```python
from build123d import *

# Parameters (mm, degrees)
EXTRUDE_THIN1_DEPTH = 9.525
FILLET1_R           = 1
FILLET3_R           = 2
FILLET4_R           = 2
SKETCH2_R           = 2.2
CUT_EXTRUDE1_DEPTH  = 23.468607993
CUT_EXTRUDE2_REACH  = 24.469
SKETCH3_R           = 1.7525


with BuildPart() as part:
    # Sketch1 → Extrude-Thin1 (new body)
    with BuildSketch(Plane(origin=(0, 0, 0), x_dir=(1, 0, 0), z_dir=(0, 1, 0))):
        Polygon((0, 0), (0, -15.9004), (12.7, -15.9004), (12.7, 0), (11.1125, 0), (11.1125, -14.3129), (1.5875, -14.3129), (1.5875, 0), align=None)
    extrude(amount=EXTRUDE_THIN1_DEPTH)

    # Fillet1
    fillet1_edges = [part.edges().sort_by_distance(p)[0] for p in [
        (1.5875, 4.7625, 14.3129),
        (11.1125, 4.7625, 14.3129),
    ]]
    fillet(fillet1_edges, radius=FILLET1_R)

    # Fillet3
    fillet3_edges = [part.edges().sort_by_distance(p)[0] for p in [
        (12.7, 4.7625, 15.9004),
        (0, 4.7625, 15.9004),
    ]]
    fillet(fillet3_edges, radius=FILLET3_R)

    # Fillet4
    fillet4_edges = [part.edges().sort_by_distance(p)[0] for p in [
        (0.79375, 9.525, 0),
        (0.79375, 0, 0),
        (11.90625, 9.525, 0),
        (11.90625, 0, 0),
    ]]
    fillet(fillet4_edges, radius=FILLET4_R)

    # Sketch2 → Cut-Extrude1 (cut, through all)
    with BuildSketch(Plane.ZY):
        with Locations((4.7625, 4.7625)):
            Circle(SKETCH2_R)
    extrude(amount=-CUT_EXTRUDE1_DEPTH, mode=Mode.SUBTRACT)

    # Sketch3 → Cut-Extrude2 (cut, up to next)
    with BuildSketch(Plane.XY.offset(15.9004), mode=Mode.PRIVATE) as cut_extrude2_sk1:
        with Locations((6.35, 4.7625)):
            Circle(SKETCH3_R)
    cut_extrude2_tool1 = extrude(cut_extrude2_sk1.sketch, amount=-CUT_EXTRUDE2_REACH, mode=Mode.PRIVATE) & part.part
    add(cut_extrude2_tool1.solids().sort_by_distance((6.35, 4.7625, 15.9004))[0], mode=Mode.SUBTRACT)


solid = part.part
```
Here's how the part is built. I have some questions about the finished solid (model axes, mm). A direction names the side the tool comes from. Coordinates: 2 decimals unless noted, no trailing zeros. Order: outer loops, then holes, each group sorted by start corner. A loop starts at its lowest first (then second) coordinate and runs counter-clockwise, first axis right, second up.
Item 1: If we section it at B-B, the plane z = 9.5: List the corners of the cut face in (x, y) for me (1 decimal), then the cut area to 3 significant figures.
Response values:
outline: (0, 0) - (1.6, 0) - (1.6, 9.5) - (0, 9.5) - close; (11.1, 0) - (12.7, 0) - (12.7, 9.5) - (11.1, 9.5) - close
area: 30.2 mm2
Item 2: Thinking about a two-plate mould opening in Y: for faces 3 (the face through (6, 9.525, 15)), 4 (the face through (1.89, 4.83, 14.03)), 5 (the face through (5.97, 3.05, 15.12)), which applies, pulls with the +Y half, pulls with the -Y half, needs draft (parallel to the pull), parting line crosses it, or undercut?
Response values:
face 3: pulls with the +Y half
face 4: needs draft
face 5: undercut
Item 3: If we section it at A-A, the plane x = 6.35: List the corners of the cut face in (y, z) for me (3 decimals), then the cut area to 3 significant figures.
Response values:
outline: (0, 14.313) - (3.01, 14.313) - (3.01, 15.9) - (0, 15.9) - close; (6.515, 14.313) - (9.525, 14.313) - (9.525, 15.9) - (6.515, 15.9) - close
area: 9.56 mm2
Item 4: I'm going to push a flat-ended pin straight in: pin 1 Ø4 at (x, y) = (6.5, 4) entering from -Z. Where does the tip first touch, or does it pass through?
Response values:
pin 1: stops at z = 14.31
Item 5: I need wall thicknesses on probe 1 along X at (y, z) = (6.25, 13.25); probe 2 along Z at (x, y) = (4.5, 3); probe 3 along Z at (x, y) = (12, 3.75). Which ranges of each line are inside material? Lowest first, please.
Response values:
probe 1: x = 0 to 1.59, 11.11 to 12.7
probe 2: z = 14.31 to 15.9
probe 3: z = 0 to 2.81, 6.72 to 15.42
Item 6: Which directions (+Z, -Z, +X, -X, +Y, -Y) give clear straight access to the entire face, cutting with the end or side of a thin tool? Please do faces 1 (the face through (1, 5, 0)), 2 (the face through (10.83, 4.83, 14.01)).
Response values:
face 1: -Z, +X, -X, +Y, -Y
face 2: -Z, +Y, -Y
Item 7: If we section it at D-D, the plane z = 5: List the corners of the cut face in (x, y) for me (1 decimal), then the cut area to 3 significant figures.
Response values:
outline: (0, 0) - (1.6, 0) - (1.6, 2.6) - (0, 2.6) - close; (0, 6.9) - (1.6, 6.9) - (1.6, 9.5) - (0, 9.5) - close; (11.1, 0) - (12.7, 0) - (12.7, 2.6) - (11.1, 2.6) - close; (11.1, 6.9) - (12.7, 6.9) - (12.7, 9.5) - (11.1, 9.5) - close
area: 16.4 mm2
Item 8: If we section it at C-C, the plane y = 3.25: List the corners of the cut face in (x, z) for me.
Response values:
outline: (0, 0) - (1.59, 0) - (1.59, 3.16) - (0, 3.16) - close; (0, 6.36) - (1.59, 6.36) - (1.59, 13.31) arc R1 cw to (2.59, 14.31) - (5.46, 14.31) - (5.46, 15.9) - (2, 15.9) arc R2 ccw to (0, 13.9) - close; (7.24, 14.31) - (10.11, 14.31) arc R1 cw to (11.11, 13.31) - (11.11, 6.36) - (12.7, 6.36) - (12.7, 13.9) arc R2 ccw to (10.7, 15.9) - (7.24, 15.9) - close; (11.11, 0) - (12.7, 0) - (12.7, 3.16) - (11.11, 3.16) - close
